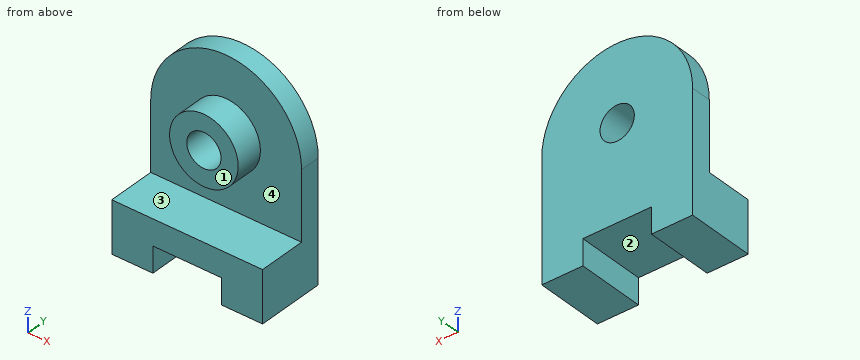
from build123d import *

# Parameters (mm, degrees)
F1_DEPTH = 40
F0_R     = 20
F2_DEPTH = 12
F0_R_2   = 10
F3_DEPTH = 28


with BuildPart() as f1:
    # F0 (on Front) → F1 (new body)
    with BuildSketch(Plane.XZ):
        Polygon((-20, -55), (0, -55), (20, -55), (20, -70), (44, -70), (44, -40), (0, -40), (-44, -40), (-44, -70), (-20, -70), align=None)
    extrude(amount=F1_DEPTH)

    # F0 (on Front) → F2 (join)
    with BuildSketch(Plane.XZ):
        Polygon((-20, -55), (0, -55), (20, -55), (20, -70), (44, -70), (44, -40), (0, -40), (-44, -40), (-44, -70), (-20, -70), align=None)
        with BuildLine():
            Line((-44, 0), (-44, -40))
            Line((-44, -40), (0, -40))
            Line((0, -40), (44, -40))
            Line((44, -40), (44, 0))
            ThreePointArc((44, 0), (0, 44), (-44, 0))
        make_face()
        Circle(F0_R, mode=Mode.SUBTRACT)
    extrude(amount=F2_DEPTH)

    # F0 (on Front) → F3 (join)
    with BuildSketch(Plane.XZ):
        Circle(F0_R)
        Circle(F0_R_2, mode=Mode.SUBTRACT)
    extrude(amount=F3_DEPTH)


solid = f1.part
Source: CAD feature listing. Evaluate the final solid. Frame: model axes, mm. Face numbers are marked on the shaded views. A direction names the side the tool comes from. Round coordinates to 2 decimals unless told otherwise and drop trailing zeros. Order: outer loops, then holes, each group sorted by start corner. A loop starts at its lowest first (then second) coordinate and runs counter-clockwise, first axis right, second up. Notation, with made-up numbers: (-18, 70.25) -> (-10, 70.25) arc R24 ccw to (-10, 93.25) -> close; hole circle Ø5 at (23.5, -34). An arc over 180 degrees is marked (long way). Answer as CSV lines item,"result".
Item 1: Section A-A, the plane y = -23. Return loops of the section in (x, z), plus the area to 3 significant figures.
A:
outline,"(-44, -70) -> (-20, -70) -> (-20, -55) -> (20, -55) -> (20, -70) -> (44, -70) -> (44, -40) -> (-44, -40) -> close; circle Ø40 at (0, 0); hole circle Ø20 at (0, 0)"
area,"2,980 mm²"
Item 2: Line query: L1, parallel to Z at x = 0, y = -20.5; L2, parallel to Z at x = 0, y = -11.5; L3, parallel to X at y = -29.5, z = -62. Output: solid intervals per line, ascending.
A:
L1,"-55 to -40, -20 to -10, 10 to 20"
L2,"-55 to -10, 10 to 44"
L3,"-44 to -20, 20 to 44"
Item 3: Section D-D, the plane y = -3.5. Return loops of the section in (x, z).
A:
outline,"(-44, -70) -> (-20, -70) -> (-20, -55) -> (20, -55) -> (20, -70) -> (44, -70) -> (44, 0) arc R44 ccw to (-44, 0) -> close; hole circle Ø20 at (0, 0)"
Item 4: Pin query (flat end, axial travel): pin 1 Ø6 at (x, z) = (3, -30) entering from -Y; pin 2 Ø3 at (x, y) = (-15.5, -17) entering from +Z; pin 3 Ø2 at (x, z) = (9, -10) entering from -Y. Return the tip coordinate at first contact, or that it passes through.
A:
pin 1,"y = -12"
pin 2,"z = 14.28"
pin 3,"y = -28"
Item 5: Section C-C, the plane z = -16. Return loops of the section in (x, y), plus the area to 3 significant figures.
A:
outline,"(-44, -12) -> (-12, -12) -> (-12, -28) -> (12, -28) -> (12, -12) -> (44, -12) -> (44, 0) -> (-44, 0) -> close"
area,"1,440 mm²"
Item 6: Reachability of the marked faces 1, 2, 3 and 4 from +Z, -Z, +X, -X, +Y, -Y: full face, straight path, thin tool, end or side. Return the list, or none.
A:
face 1,"+Z, +X, -X, -Y"
face 2,"-Z, +Y, -Y"
face 3,"+X, -X, -Y"
face 4,"-Y"
Item 7: Section B-B, the plane x = 0. Return loops of the section in (y, z).
A:
outline,"(-40, -55) -> (0, -55) -> (0, -10) -> (-28, -10) -> (-28, -20) -> (-12, -20) -> (-12, -40) -> (-40, -40) -> close; (-28, 10) -> (0, 10) -> (0, 44) -> (-12, 44) -> (-12, 20) -> (-28, 20) -> close"
